```python
from build123d import *

# Parameters (mm, degrees)
PAD_DEPTH       = 46.5
SKETCH114_W     = 3
SKETCH114_H     = 2
SKETCH114_W_2   = 1
SKETCH114_H_2   = 3
POCKET_DEPTH    = 46.501
SKETCH116_R     = 14.23
SKETCH116_R_2   = 1.5
POCKET001_DEPTH = 5
SKETCH_W        = 2
SKETCH_H        = 35
POCKET002_DEPTH = 7
POCKET003_START = 7
SKETCH117_W     = 2
SKETCH117_H     = 3
SKETCH117_W_2   = 3
SKETCH117_H_2   = 1
POCKET003_DEPTH = 40
PAD001_START    = -4
SKETCH119_W     = 1.5
SKETCH119_H     = 3
SKETCH119_W_2   = 2.5
SKETCH119_H_2   = 0.9
PAD001_DEPTH    = 85
SKETCH118_R     = 1.25
SKETCH118_W     = 12
SKETCH118_H     = 6
POCKET004_DEPTH = 94.001
SKETCH120_W     = 13.5
SKETCH120_H     = 6
POCKET005_DEPTH = 5


with BuildPart() as part:
    # Sketch112 → Pad (new body)
    with BuildSketch(Plane.XY):
        with BuildLine():
            Line((0, 0), (-89, 0))
            ThreePointArc((-94, 5), (-92.535534, 1.464466), (-89, 0))
            Line((-94, 5), (-94, 45))
            Line((-94, 45), (-90, 45))
            Line((-90, 5), (-90, 45))
            ThreePointArc((-90, 5), (-89.707107, 4.292893), (-89, 4))
            Line((0, 4), (-89, 4))
            Line((0, 4), (0, 0))
        make_face()
    extrude(amount=PAD_DEPTH)

    # Sketch114 → Pocket (cut, through all)
    with BuildSketch(Plane.XY):
        with Locations((-1.5, 2)):
            Rectangle(SKETCH114_W, SKETCH114_H)
        with Locations((-3.5, 2)):
            Rectangle(SKETCH114_W_2, SKETCH114_H_2)
    extrude(amount=POCKET_DEPTH, mode=Mode.SUBTRACT)

    # Sketch116 → Pocket001 (cut)
    with BuildSketch(Plane.XZ):
        with Locations((-21.95, 27)):
            Circle(SKETCH116_R)
        with Locations((-10, 38.95)):
            Circle(SKETCH116_R_2)
        with Locations((-33.9, 38.95)):
            Circle(SKETCH116_R_2)
        with Locations((-33.9, 15.05)):
            Circle(SKETCH116_R_2)
        with Locations((-10, 15.05)):
            Circle(SKETCH116_R_2)
    extrude(amount=-POCKET001_DEPTH, mode=Mode.SUBTRACT)

    # Sketch → Pocket002 (cut)
    with BuildSketch(Plane.XY):
        with Locations((-92, 27.5)):
            Rectangle(SKETCH_W, SKETCH_H)
    extrude(amount=POCKET002_DEPTH, mode=Mode.SUBTRACT)

    # Sketch117 → Pocket003 (cut)
    with BuildSketch(Plane.XY.offset(POCKET003_START)):
        with Locations((-92, 43.5)):
            Rectangle(SKETCH117_W, SKETCH117_H)
        with Locations((-92, 41.5)):
            Rectangle(SKETCH117_W_2, SKETCH117_H_2)
    extrude(amount=POCKET003_DEPTH, mode=Mode.SUBTRACT)

    # Sketch119 → Pad001 (join)
    with BuildSketch(Plane.YZ.offset(PAD001_START)):
        with Locations((2, 48)):
            Rectangle(SKETCH119_W, SKETCH119_H)
        with Locations((2, 49.95)):
            Rectangle(SKETCH119_W_2, SKETCH119_H_2)
    extrude(amount=-PAD001_DEPTH)

    # Sketch118 → Pocket004 (cut, through all)
    with BuildSketch(Plane.YZ):
        with Locations((34, 13)):
            Circle(SKETCH118_R)
        with Locations((18, 13)):
            Circle(SKETCH118_R)
        with Locations((26, 13)):
            Rectangle(SKETCH118_W, SKETCH118_H)
    extrude(amount=-POCKET004_DEPTH, mode=Mode.SUBTRACT)

    # Sketch120 → Pocket005 (cut)
    with BuildSketch(Plane.XZ):
        with Locations((-21.95, 6)):
            Rectangle(SKETCH120_W, SKETCH120_H)
    extrude(amount=-POCKET005_DEPTH, mode=Mode.SUBTRACT)


solid = part.part
```
Geometry check sheet. Reference: the model listing, model coordinates, mm. A direction names the side the tool comes from. Round coordinates to 2 decimals unless told otherwise and drop trailing zeros. Loops run counter-clockwise (first coordinate to the right, second up) from the corner with the lowest first, then second, coordinate; pieces in that order, holes last. Notation, with made-up numbers: M 4.25,-38.75 L 14.25,-38.75 A7 cw 14.25,-29.75 Z; hole C -17,-21 d6. An arc over 180 degrees is marked long. Return JSON: item names as keys, results as strings. Group by question number.
(1) Scan lines: line 1 along X through (y, z) = (41, 3); line 2 along Z through (x, y) = (-33.9, 1.35); line 3 along Z through (x, y) = (-92.1, 34). Record each from-to range of solid material in increasing order. Write a range as [from, to].
(2) Go/stop test with flat-tipped pins: pin 1 (0.5 mm diameter, centred on y = 41.5, z = 36, fed in from +X); pin 2 (1.6 mm diameter, centred on x = -92, z = 4.5, fed in from +Y); pin 3 (0.9 mm diameter, centred on x = -2, z = 20.5, fed in from +Y). Record where each tip stops, or that it passes through.
(3) Mould release check, pull along Z, two halves, no side actions. Record for faces 5 (the face through (-50, 3, 0)), 6 (the face through (-91, 33, 6)), 7 (the face through (-91.972, 34.672, 14.054)): pulls with the +Z half, pulls with the -Z half, needs draft (parallel to the pull), parting line crosses it, or undercut.
(4) Section check B-B, the plane y = 34. Enter the section's corners in (x, z), and give its area (3 significant figures).
(5) Section check A-A, the plane z = 27. Enter the section's corners in (x, y).
(6) Section check D-D, the plane x = -10. Enter the section's corners in (y, z).
(7) Section check C-C, the plane x = -71.5. Enter the section's corners in (y, z), and give its area (3 significant figures).
(8) Set-up check for faces 1 (the face through (-22, 2, 3)), 2 (the face through (-92, 26, 16)), 3 (the face through (-46, 2.75, 48)), 4 (the face through (-92, 10, 3)): record each of +Z, -Z, +X, -X, +Y, -Y from which the full face is reachable in a straight line by a thin tool's end or side.
Data:
{
 "1": {"line 1": "[-94, -93], [-91, -90]", "line 2": "[0, 13.55], [16.55, 19.27], [34.73, 37.45], [40.45, 50.4]", "line 3": "[7, 11.75], [14.25, 46.5]"},
 "2": {"pin 1": "x = -90", "pin 2": "y = 10", "pin 3": "y = 4"},
 "3": {"face 5": "pulls with the -Z half", "face 6": "needs draft", "face 7": "undercut"},
 "4": {"outline": "M -94,0 L -93,0 L -93,7 L -91,7 L -91,0 L -90,0 L -90,11.75 L -94,11.75 Z; M -94,14.25 L -90,14.25 L -90,46.5 L -94,46.5 Z", "area": "162 mm²"},
 "5": {"outline": "M -94,5 A5 ccw -89,0 L -36.18,0 L -36.18,4 L -89,4 A1 cw -90,5 L -90,45 L -91,45 L -91,42 L -90.5,42 L -90.5,41 L -93.5,41 L -93.5,42 L -93,42 L -93,45 L -94,45 Z; M -7.72,0 L 0,0 L 0,1 L -3,1 L -3,0.5 L -4,0.5 L -4,3.5 L -3,3.5 L -3,3 L 0,3 L 0,4 L -7.72,4 Z"},
 "6": {"outline": "M 0,0 L 4,0 L 4,13.55 L 0,13.55 Z; M 0,16.55 L 4,16.55 L 4,19.27 L 0,19.27 Z; M 0,34.73 L 4,34.73 L 4,37.45 L 0,37.45 Z; M 0,40.45 L 4,40.45 L 4,46.5 L 2.75,46.5 L 2.75,49.5 L 3.25,49.5 L 3.25,50.4 L 0.75,50.4 L 0.75,49.5 L 1.25,49.5 L 1.25,46.5 L 0,46.5 Z"},
 "7": {"outline": "M 0,0 L 4,0 L 4,46.5 L 2.75,46.5 L 2.75,49.5 L 3.25,49.5 L 3.25,50.4 L 0.75,50.4 L 0.75,49.5 L 1.25,49.5 L 1.25,46.5 L 0,46.5 Z", "area": "193 mm²"},
 "8": {"face 1": "+Y, -Y", "face 2": "+X, -X", "face 3": "+X, -X, +Y", "face 4": "-Z, +Y"}
}
